from build123d import *

# Parameters (mm, degrees)
F0_W     = 30
F0_H     = 30
F0_R     = 3
F1_DEPTH = 5
F2_W     = 25
F2_H     = 20
F2_R     = 9.5
F3_DEPTH = 3
F4_W     = 25
F4_H     = 20
F4_R     = 4
F5_DEPTH = 2
F6_W     = 25
F6_H     = 20
F6_R     = 6
F7_DEPTH = 5


with BuildPart() as f1:
    # F0 (on Top) → F1 (new body)
    with BuildSketch(Plane.XY):
        Rectangle(F0_W, F0_H)
        with Locations((-7, -7)):
            Circle(F0_R, mode=Mode.SUBTRACT)
        with Locations((7, -7)):
            Circle(F0_R, mode=Mode.SUBTRACT)
        with Locations((-7, 7)):
            Circle(F0_R, mode=Mode.SUBTRACT)
        Circle(F0_R, mode=Mode.SUBTRACT)
        with Locations((7, 7)):
            Circle(F0_R, mode=Mode.SUBTRACT)
    extrude(amount=F1_DEPTH)

    # F2 (on face) → F3 (join)
    with BuildSketch(Plane.YZ.offset(15)):
        with Locations((2.5, 15)):
            Rectangle(F2_W, F2_H)
        with Locations((0, 15)):
            Circle(F2_R, mode=Mode.SUBTRACT)
    extrude(amount=-F3_DEPTH)

    # F4 (on face) → F5 (join)
    with BuildSketch(Plane(origin=(12, 0, 0), x_dir=(0, -1, 0), z_dir=(-1, 0, 0))):
        with Locations((-2.5, 15)):
            Rectangle(F4_W, F4_H)
        with Locations((0, 15)):
            Circle(F4_R, mode=Mode.SUBTRACT)
    extrude(amount=F5_DEPTH)

    # F6 (on face) → F7 (join)
    with BuildSketch(Plane(origin=(0, 15, 0), x_dir=(-1, 0, 0), z_dir=(0, 1, 0))):
        with Locations((2.5, 15)):
            Rectangle(F6_W, F6_H)
        with Locations((0, 12)):
            Circle(F6_R, mode=Mode.SUBTRACT)
    extrude(amount=-F7_DEPTH)


solid = f1.part
The listing builds one solid part. Answer for the finished solid, in the listing's coordinates (mm). A direction names the side the tool comes from. Round coordinates to 2 decimals unless told otherwise and drop trailing zeros. Order: outer loops, then holes, each group sorted by start corner. A loop starts at its lowest first (then second) coordinate and runs counter-clockwise, first axis right, second up. Notation, with made-up numbers: (49.25, 33) -> (66.25, 33) arc R7 ccw to (66.25, 44) -> close; hole circle Ø2 at (78.5, -1). An arc over 180 degrees is marked (long way). Put each result on its own line as item: value.
Q1. Which of the six approach directions +Z, -Z, +X, -X, +Y, -Y give full straight-line access (tool end or side, diameter ignored) to faces 4 (the cylindrical face through (13.521, 9.061, 17.854)), 5 (the cylindrical face through (-4.14, 7.9, 2.46)), 6 (the flat face through (13, -10, 15)), 7 (the flat face through (9.3, 9.4, 5))?
Results list:
face 4: +X
face 5: +Z, -Z
face 6: +Z, +X, -X, -Y
face 7: +Z, -X, -Y
Q2. Each of these flat-tipped pins is pushed along its axis until it touches: P1, Ø1.5, axis at x = 11.5, z = 14.5, coming from the -Y side; P2, Ø5, axis at x = 6, y = -6, coming from the +Z side; P3, Ø10, axis at x = 1, z = 15, coming from the -Y side. Where does it stop, or does it pass through?
Results list:
P1: y = -10
P2: z = 5
P3: y = 10
Q3. Section A-A, the plane x = 0 is taken. Write down the section's boundary in (y, z).
Results list:
outline: (-15, 0) -> (-3, 0) -> (-3, 5) -> (-15, 5) -> close; (3, 0) -> (15, 0) -> (15, 6) -> (10, 6) -> (10, 5) -> (3, 5) -> close; (10, 18) -> (15, 18) -> (15, 25) -> (10, 25) -> close
Q4. Section D-D, the plane y = -4.5 is taken. Write down the section's boundary in (x, z).
Results list:
outline: (-15, 0) -> (-8.66, 0) -> (-8.66, 5) -> (-15, 5) -> close; (-5.34, 0) -> (5.34, 0) -> (5.34, 5) -> (-5.34, 5) -> close; (8.66, 0) -> (15, 0) -> (15, 6.63) -> (12, 6.63) -> (12, 23.37) -> (15, 23.37) -> (15, 25) -> (10, 25) -> (10, 5) -> (8.66, 5) -> close
Q5. Consider line 1 along Y through (x, z) = (-7, 4); line 2 along Z through (x, y) = (-3.75, 1). Determine where each line is inside the solid, lowest interval first.
Results list:
line 1: -15 to -10, -4 to 4, 10 to 15
line 2: 0 to 5
Q6. Section B-B, the plane z = 3.75 is taken. Write down the section's boundary in (x, y).
Results list:
outline: (-15, -15) -> (15, -15) -> (15, 15) -> (-15, 15) -> close; hole circle Ø6 at (-7, -7); hole circle Ø6 at (-7, 7); hole circle Ø6 at (0, 0); hole circle Ø6 at (7, -7); hole circle Ø6 at (7, 7)
Q7. Determine the mould class of faces 1 (the flat face through (0, -15, 2)), 2 (the flat face through (-15, 7, 4)), 3 (the cylindrical face through (-4.14, -6.1, 2.46)) for opening direction X: pulls with the +X half, pulls with the -X half, needs draft (parallel to the pull), parting line crosses it, or undercut.
Results list:
face 1: needs draft
face 2: pulls with the -X half
face 3: undercut
Q8. Section C-C, the plane z = 9 is taken. Write down the section's boundary in (x, y), and give its area (3 significant figures).
Results list:
outline: (-15, 10) -> (-5.2, 10) -> (-5.2, 15) -> (-15, 15) -> close; (5.2, 10) -> (10, 10) -> (10, -10) -> (15, -10) -> (15, -7.37) -> (12, -7.37) -> (12, 7.37) -> (15, 7.37) -> (15, 15) -> (5.2, 15) -> close
area: 154 mm^2
